Geometry check sheet. Reference: drawing and pictorial views, mm from the part's lowest x, y, z. A direction names the side the tool comes from. Give positions to 0.01 mm unless a question says otherwise; leave off trailing zeros. Order: outer loops, then holes, each group sorted by start corner. A loop starts at its lowest first (then second) coordinate and runs counter-clockwise, first axis right, second up.
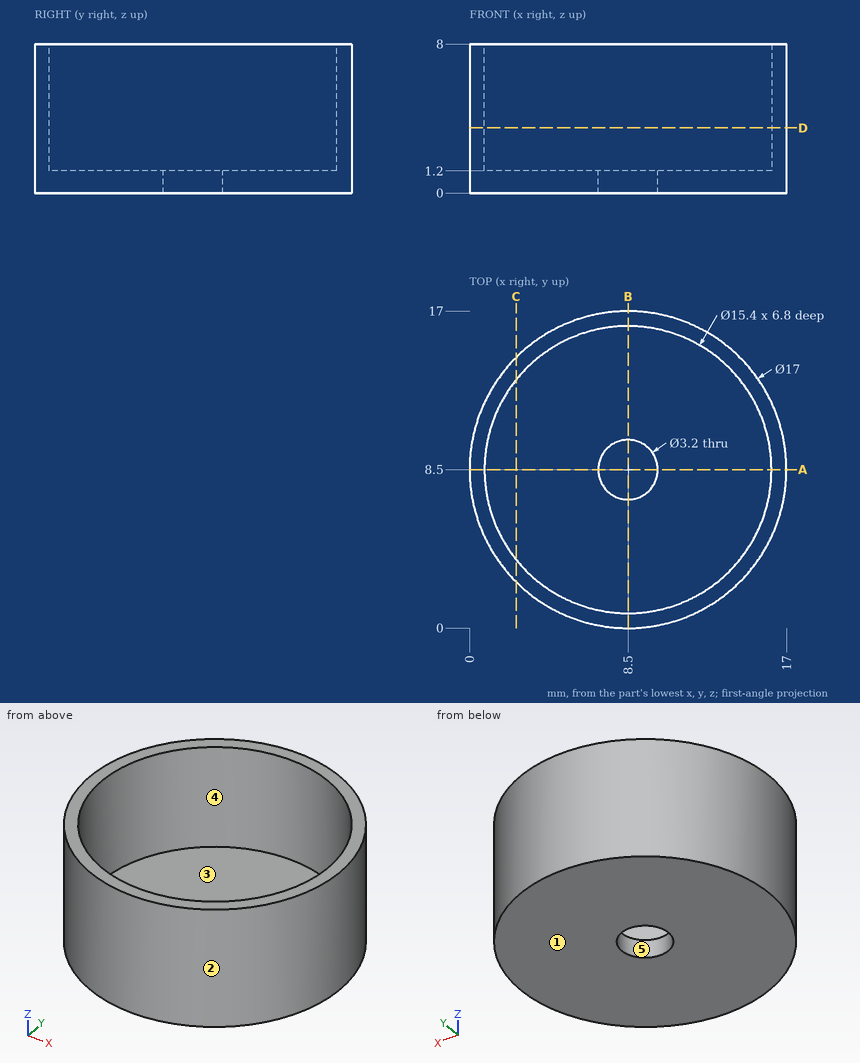
(1) Sectioned sample at D-D (z = 3.5). Enter the section's corners in (x, y).
(2) Thickness scan on L1, parallel to Y at x = 8.25, z = 5.25; L2, parallel to Y at x = 8.5, z = 0.5; L3, parallel to Z at x = 10, y = 14.5. Record the ranges inside material, lowest first.
(3) Release check for a two-part mould opening along X. For the marked faces 1, 2 and 3 record: released by +X, released by -X, zero draft, split by the parting line, or undercut.
(4) Go/stop test with flat-tipped pins: P1, Ø4.5, axis at x = 12, y = 10.5, coming from the +Z side; P2, Ø1.5, axis at x = 6.5, z = 4.5, coming from the -Y side; P3, Ø3, axis at x = 8.5, y = 8.5, coming from the +Z side; P4, Ø1.5, axis at x = 12, z = 2.5, coming from the -Y side. Record where each tip stops, or that it passes through.
(5) Sectioned sample at A-A (y = 8.5). Enter the section's corners in (x, z), plus the area to 3 significant figures.
(6) Tool access check on the marked faces 4 and 5. Record the directions out of +Z, -Z, +X, -X, +Y, -Y that give a thin tool (end or side, any length) a straight path to the whole face; none if there is none.
(7) Sectioned sample at C-C (x = 2.5). Enter the section's corners in (y, z).
Values follow:
1. outline: circle Ø17 at (8.5, 8.5); hole circle Ø15.4 at (8.5, 8.5)
2. L1: y = 0 to 0.8, 16.2 to 17
2. L2: y = 0 to 6.9, 10.1 to 17
2. L3: z = 0 to 1.2
3. face 1: zero draft
3. face 2: split by the parting line
3. face 3: undercut
4. P1: stops at z = 1.2
4. P2: stops at y = 0.09
4. P3: passes through
4. P4: stops at y = 0.46
5. outline: (0, 0) - (6.9, 0) - (6.9, 1.2) - (0.8, 1.2) - (0.8, 8) - (0, 8) - close; (10.1, 0) - (17, 0) - (17, 8) - (16.2, 8) - (16.2, 1.2) - (10.1, 1.2) - close
5. area: 27.4 mm2
6. face 4: +Z
6. face 5: +Z, -Z
7. outline: (2.48, 0) - (14.52, 0) - (14.52, 8) - (13.33, 8) - (13.33, 1.2) - (3.67, 1.2) - (3.67, 8) - (2.48, 8) - close
